from build123d import *

# Parameters (mm, degrees)
F0_W     = 28
F0_H     = 0.3
F0_W_2   = 28.3
F0_H_2   = 0.2
F0_H_3   = 0.1
F0_W_3   = 0.3
F1_DEPTH = 10
F1_TAPER = -10


with BuildPart() as f1:
    # F0 (on Top) → F1 (new body)
    with BuildSketch(Plane.XY):
        Polygon((28, 0), (0, 0), (0, 25), (28, 25), (28, 25.1), (-0.3, 25.1), (-0.3, -0.3), (28, -0.3), align=None)
        with Locations((42.3, -0.15)):
            Rectangle(F0_W, F0_H)
        with Locations((13.85, 25.2)):
            Rectangle(F0_W_2, F0_H_2)
        with Locations((13.85, 50.6)):
            Rectangle(F0_W_2, F0_H_2)
        Polygon((-0.3, 101.5), (-0.3, 76.1), (28, 76.1), (28, 76.2), (0, 76.2), (0, 101.2), (28, 101.2), (28, 101.5), align=None)
        with Locations((13.85, 76)):
            Rectangle(F0_W_2, F0_H_2)
        with Locations((42.3, 101.35)):
            Rectangle(F0_W, F0_H)
        with Locations((70.6, -0.15)):
            Rectangle(F0_W, F0_H)
        with Locations((70.6, 101.35)):
            Rectangle(F0_W, F0_H)
        Polygon((84.9, 0), (84.9, -0.3), (113.2, -0.3), (113.2, 25.1), (84.9, 25.1), (84.9, 25), (112.9, 25), (112.9, 0), align=None)
        with Locations((99.05, 25.2)):
            Rectangle(F0_W_2, F0_H_2)
        with Locations((99.05, 50.6)):
            Rectangle(F0_W_2, F0_H_2)
        with Locations((99.05, 76)):
            Rectangle(F0_W_2, F0_H_2)
        Polygon((84.9, 76.1), (113.2, 76.1), (113.2, 101.5), (84.9, 101.5), (84.9, 101.2), (112.9, 101.2), (112.9, 76.2), (84.9, 76.2), align=None)
        Polygon((-0.3, 25.3), (28, 25.3), (28, 25.4), (0, 25.4), (0, 50.4), (28, 50.4), (28, 50.5), (-0.3, 50.5), align=None)
        Polygon((-0.3, 75.9), (-0.3, 50.7), (28, 50.7), (28, 50.8), (0, 50.8), (0, 75.8), (28, 75.8), (28, 75.9), align=None)
        Polygon((84.9, 25.4), (84.9, 25.3), (113.2, 25.3), (113.2, 50.5), (84.9, 50.5), (84.9, 50.4), (112.9, 50.4), (112.9, 25.4), align=None)
        Polygon((84.9, 50.7), (113.2, 50.7), (113.2, 75.9), (84.9, 75.9), (84.9, 75.8), (112.9, 75.8), (112.9, 50.8), (84.9, 50.8), align=None)
        Polygon((28, 25), (28, 0), (28, -0.3), (28.3, -0.3), (28.3, 0), (28.3, 25), (28.3, 25.1), (28, 25.1), align=None)
        Polygon((28, 76.2), (28, 76.1), (28.3, 76.1), (28.3, 76.2), (28.3, 101.2), (28.3, 101.5), (28, 101.5), (28, 101.2), align=None)
        Polygon((84.6, 0), (84.6, -0.3), (84.9, -0.3), (84.9, 0), (84.9, 25), (84.9, 25.1), (84.6, 25.1), (84.6, 25), align=None)
        Polygon((84.6, 76.2), (84.6, 76.1), (84.9, 76.1), (84.9, 76.2), (84.9, 101.2), (84.9, 101.5), (84.6, 101.5), (84.6, 101.2), align=None)
        Polygon((56.3, 0), (56.3, -0.3), (56.6, -0.3), (56.6, 0), (56.6, 25), (56.6, 25.1), (56.3, 25.1), (56.3, 25), align=None)
        Polygon((56.3, 76.2), (56.3, 76.1), (56.6, 76.1), (56.6, 76.2), (56.6, 101.2), (56.6, 101.5), (56.3, 101.5), (56.3, 101.2), align=None)
        with Locations((42.3, 25.35)):
            Rectangle(F0_W, F0_H_3)
        with Locations((70.6, 25.35)):
            Rectangle(F0_W, F0_H_3)
        Polygon((28, 25.4), (28, 25.3), (28.3, 25.3), (28.3, 25.4), (28.3, 50.4), (28.3, 50.5), (28, 50.5), (28, 50.4), align=None)
        Polygon((28, 50.8), (28, 50.7), (28.3, 50.7), (28.3, 50.8), (28.3, 75.8), (28.3, 75.9), (28, 75.9), (28, 75.8), align=None)
        with Locations((42.3, 25.2)):
            Rectangle(F0_W, F0_H_2)
        with Locations((70.6, 25.05)):
            Rectangle(F0_W, F0_H_3)
        with Locations((70.6, 50.75)):
            Rectangle(F0_W, F0_H_3)
        with Locations((70.6, 75.85)):
            Rectangle(F0_W, F0_H_3)
        with Locations((42.3, 50.6)):
            Rectangle(F0_W, F0_H_2)
        with Locations((42.3, 75.85)):
            Rectangle(F0_W, F0_H_3)
        Polygon((84.6, 25.4), (84.6, 25.3), (84.9, 25.3), (84.9, 25.4), (84.9, 50.4), (84.9, 50.5), (84.6, 50.5), (84.6, 50.4), align=None)
        Polygon((84.6, 50.8), (84.6, 50.7), (84.9, 50.7), (84.9, 50.8), (84.9, 75.8), (84.9, 75.9), (84.6, 75.9), (84.6, 75.8), align=None)
        with Locations((42.3, 25.05)):
            Rectangle(F0_W, F0_H_3)
        with Locations((70.6, 25.2)):
            Rectangle(F0_W, F0_H_2)
        Polygon((56.3, 25.4), (56.3, 25.3), (56.6, 25.3), (56.6, 25.4), (56.6, 50.4), (56.6, 50.5), (56.3, 50.5), (56.3, 50.4), align=None)
        Polygon((56.3, 50.8), (56.3, 50.7), (56.6, 50.7), (56.6, 50.8), (56.6, 75.8), (56.6, 75.9), (56.3, 75.9), (56.3, 75.8), align=None)
        with Locations((70.6, 50.6)):
            Rectangle(F0_W, F0_H_2)
        with Locations((42.3, 50.45)):
            Rectangle(F0_W, F0_H_3)
        with Locations((70.6, 76)):
            Rectangle(F0_W, F0_H_2)
        with Locations((42.3, 76)):
            Rectangle(F0_W, F0_H_2)
        with Locations((70.6, 76.15)):
            Rectangle(F0_W, F0_H_3)
        with Locations((42.3, 76.15)):
            Rectangle(F0_W, F0_H_3)
        with Locations((42.3, 50.75)):
            Rectangle(F0_W, F0_H_3)
        with Locations((70.6, 50.45)):
            Rectangle(F0_W, F0_H_3)
        with Locations((84.75, 76)):
            Rectangle(F0_W_3, F0_H_2)
        with Locations((56.45, 76)):
            Rectangle(F0_W_3, F0_H_2)
        with Locations((28.15, 76)):
            Rectangle(F0_W_3, F0_H_2)
        with Locations((84.75, 25.2)):
            Rectangle(F0_W_3, F0_H_2)
        with Locations((84.75, 50.6)):
            Rectangle(F0_W_3, F0_H_2)
        with Locations((28.15, 50.6)):
            Rectangle(F0_W_3, F0_H_2)
        with Locations((56.45, 50.6)):
            Rectangle(F0_W_3, F0_H_2)
        with Locations((56.45, 25.2)):
            Rectangle(F0_W_3, F0_H_2)
        with Locations((28.15, 25.2)):
            Rectangle(F0_W_3, F0_H_2)
    extrude(amount=F1_DEPTH, taper=F1_TAPER)


solid = f1.part
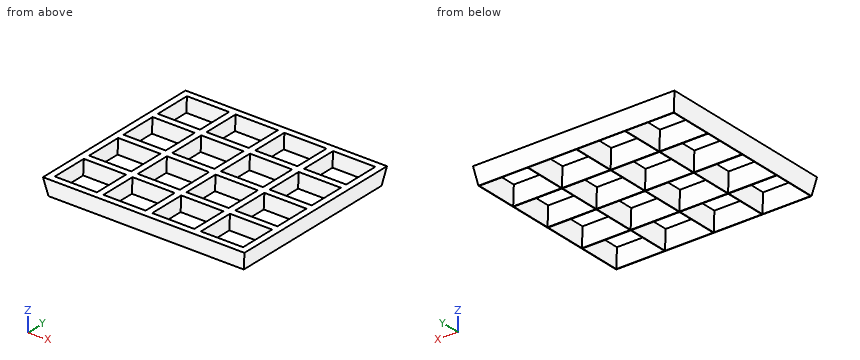
Verification items for the finished model (mm, model axes). Give positions to 0.01 mm unless a question says otherwise; leave off trailing zeros.
1) Depth check by flat-ended pin: pin 1 Ø3 at (y, z) = (49, 6.5) entering from +X; pin 2 Ø8 at (x, y) = (34.5, 37) entering from -Z; pin 3 Ø1 at (y, z) = (23, 5) entering from +X; pin 4 Ø4 at (y, z) = (74.5, 1) entering from +X. Enter the tip coordinate at first touch or a pass-through.
2) Sectioned sample at A-A, the plane y = 54.5. Count the separate pieces of the cut face and the enclosed holes in it, then the cut area to 3 significant figures.
3) Thickness scan on line 1 along Y through (x, z) = (86, 3.5); line 2 along Y through (x, z) = (24, 6.25); line 3 along X through (y, z) = (69.5, 1.75). Record the ranges inside material, lowest first.
Answers:
1. pin 1: stops at x = 114.61
1. pin 2: passes through
1. pin 3: stops at x = 114.17
1. pin 4: stops at x = 113.73
2. separate pieces: 5
2. enclosed holes: 0
2. area: 103 mm2
3. line 1: y = -0.92 to 0.62, 24.38 to 26.02, 49.78 to 51.42, 75.18 to 76.82, 100.58 to 102.12
3. line 2: y = -1.4 to 1.1, 23.9 to 26.5, 49.3 to 51.9, 74.7 to 77.3, 100.1 to 102.6
3. line 3: x = -0.61 to 0.31, 27.69 to 28.61, 55.99 to 56.91, 84.29 to 85.21, 112.59 to 113.51
